Read the model definition and answer for the solid it produces. Units are mm, in the model's axes. A direction names the side the tool comes from. Give positions to 0.01 mm unless a question says otherwise; leave off trailing zeros. Order: outer loops, then holes, each group sorted by start corner. A loop starts at its lowest first (then second) coordinate and runs counter-clockwise, first axis right, second up. Notation, with made-up numbers: (26.5, 43) - (35.5, 43) arc R25 cw to (35.5, 62) - close; hole circle Ø5 at (78.5, 66.25). An arc over 180 degrees is marked (long way). Write each question's results on one line, items separated by ' | '.
Autodesk Inventor part; units mm, degrees
ref_plane "YZ Plane" through (0, 0, 0) normal (1, 0, 0) x (0, 1, 0)
ref_plane "XZ Plane" through (0, 0, 0) normal (0, 1, 0) x (-1, 0, 0)
ref_plane "XY Plane" through (0, 0, 0) normal (0, 0, 1) x (1, 0, 0)
sketch "スケッチ1" plane through (0, 0, 0) normal (0, 0, 1) x (1, 0, 0)
  line L0 (0, 0) -> (10, 0)
  line L1 (10, 0) -> (10, 10)
  line L2 (10, 10) -> (0, 10)
  line L3 (0, 10) -> (0, 0)
  line L4 (1, 9) -> (9, 9)
  line L5 (9, 9) -> (9, 1)
  line L6 (9, 1) -> (1, 1)
  line L7 (1, 1) -> (1, 9)
  dimension "d0" = 10
  dimension "d1" = 10
  dimension "d2" = 1
extrude "押し出し1" add sketch "スケッチ1" along normal blind 52
sketch "スケッチ2" plane through (0, 10, 0) normal (0, 1, 0) x (1, 0, 0)
  line L0 (10, -52) -> (0, -52)
  line L1 (10, 0) -> (10, -52)
  line L2 (10, -26) -> (0, -26)
  line L3 (0, 0) -> (0, -52)
  point P0 (5, -37)
  point P1 (5, -14.6)
  point P2 (5, -5)
  dimension "d5" = 22.4
  dimension "d7" = 5
  dimension "d8" = 5
  dimension "d35" = 9.6
  dimension "d36" = 11
hole "穴1" at (5, 10, 37) at (5, 10, 14.6) at (5, 10, 5) direction (0, -1, 0) diameter 3 end through all
sketch "スケッチ3" plane through (10, 0, 0) normal (1, 0, 0) x (0, 0, -1)
  line L0 (0, 0) -> (-52, 0)
  line L1 (-52, 0) -> (-52, 10)
  line L2 (0, 0) -> (-52, 0)
  line L3 (-26, 0) -> (-26, 10)
  line L4 (0, 10) -> (-52, 10)
  point P0 (-31, 5)
  point P1 (-21, 5)
  dimension "d32" = 5
  dimension "d33" = 5
hole "穴2" at (10, 5, 31) at (10, 5, 21) direction (-1, 0, 0) diameter 3 end through all
sketch "スケッチ4" plane through (0, 10, 0) normal (0, 1, 0) x (1, 0, 0)
  line L0 (4.6245, -45.4744) -> (6.8253, -45.4744) construction
  line L1 (6.8253, -45.4744) -> (6.8253, -52.8345) construction
  line L2 (6.8253, -52.8345) -> (4.6245, -52.8345) construction
  line L3 (4.6245, -52.8345) -> (4.6245, -45.4744) construction
  point P0 (0, 0)
properties part number "finger_k_mk_2" material "アルミニウム 6061-AHC"
(1) Section D-D (x = 5) is taken. State how many separate pieces and enclosed holes the cut face has, plus the area to 3 significant figures.
Conclusion:
separate pieces: 8 | enclosed holes: 0 | area: 86.0 mm^2
(2) Section C-C (y = 5) is taken. Give the vertices of the cut face in (x, z), plus the area to 3 significant figures.
Conclusion:
outline: (0, 0) - (1, 0) - (1, 19.5) - (0, 19.5) - close; (0, 22.5) - (1, 22.5) - (1, 29.5) - (0, 29.5) - close; (0, 32.5) - (1, 32.5) - (1, 52) - (0, 52) - close; (9, 0) - (10, 0) - (10, 19.5) - (9, 19.5) - close; (9, 22.5) - (10, 22.5) - (10, 29.5) - (9, 29.5) - close; (9, 32.5) - (10, 32.5) - (10, 52) - (9, 52) - close | area: 92.0 mm^2
(3) Section A-A (x = 8.5) is taken. Give the vertices of the cut face in (y, z).
Conclusion:
outline: (0, 0) - (1, 0) - (1, 52) - (0, 52) - close; (9, 0) - (10, 0) - (10, 52) - (9, 52) - close
(4) Section B-B (z = 37) is taken. Give the vertices of the cut face in (x, y).
Conclusion:
outline: (0, 0) - (3.5, 0) - (3.5, 1) - (1, 1) - (1, 9) - (3.5, 9) - (3.5, 10) - (0, 10) - close; (6.5, 0) - (10, 0) - (10, 10) - (6.5, 10) - (6.5, 9) - (9, 9) - (9, 1) - (6.5, 1) - close
(5) Consider probe 1 along Z at (x, y) = (5, 0.65); probe 2 along Z at (x, y) = (0.4, 5); probe 3 along X at (y, z) = (7.75, 37.5). Determine where each line is inside the solid, lowest interval first. Write a range as [from, to].
Conclusion:
probe 1: [0, 3.5], [6.5, 13.1], [16.1, 35.5], [38.5, 52] | probe 2: [0, 19.5], [22.5, 29.5], [32.5, 52] | probe 3: [0, 1], [9, 10]
(6) The mould has two halves that part along Y. Classify faces 1 (the face through (5, 0, 26)), 2 (the face through (10, 5, 26)), 3 (the face through (5, 9, 26)), 4 (the face through (5, 10, 26)): pulls with the +Y half, pulls with the -Y half, needs draft (parallel to the pull), parting line crosses it, or undercut.
Conclusion:
face 1: pulls with the -Y half | face 2: needs draft | face 3: undercut | face 4: pulls with the +Y half
(7) For faces 5 (the face through (4.93, 9.49, 13.1)), 6 (the face through (1, 5, 26)), determine the directions among +Z, -Z, +X, -X, +Y, -Y from which every point of the face is accessible in a straight line to the end or side of a thin tool.
Conclusion:
face 5: +Y, -Y | face 6: +Z, -Z
